from build123d import *

# Parameters (mm, degrees)
SKETCH1_W   = 40
SKETCH1_H   = 40
SKETCH1_W_2 = 32
SKETCH1_H_2 = 32


with BuildPart() as part:
    # Sweep1: sweep along a curve in space
    with BuildLine() as sweep1_path:
        add(Edge.make_bspline(
            [(0, 0, -520), (0, 0, 520)],
            knots=[0, 0, 1, 1], degree=1))
    # Sketch1 → Sweep1 (sweep)
    with BuildSketch(Plane.XY):
        Rectangle(SKETCH1_W, SKETCH1_H)
        Rectangle(SKETCH1_W_2, SKETCH1_H_2, mode=Mode.SUBTRACT)
    sweep(path=sweep1_path.line)


solid = part.part
Design review of the part built by this model. Coordinates are the model's own, in mm. A direction names the side the tool comes from. Round coordinates to 2 decimals unless told otherwise and drop trailing zeros. Loops run counter-clockwise (first coordinate to the right, second up) from the corner with the lowest first, then second, coordinate; pieces in that order, holes last. Notation, with made-up numbers: (55.5, 39.25) -> (70.5, 39.25) arc R29 cw to (70.5, 59.25) -> close; hole circle Ø11 at (9, 45.5). An arc over 180 degrees is marked (long way). Use one line per item in the form item = value. Start each with the question number.
Q1. We need section C-C on z = -377.5. Give the boundary of the cut face in (x, y).
Q2. For pin 1 Ø12 at (x, y) = (12, 13.5) entering from +Z, flat-tipped, find the tip position at first contact; note if it passes through.
Q3. Wall thickness on line 1 along Y through (x, z) = (5, 251): over which ranges is the line inside the solid? List them lowest first. Write a range as [from, to].
Q4. Draft analysis for pull direction Y (two halves, no side actions). For faces 3 (the face through (0, -16, 7)), 4 (the face through (-18, 0, -520)), 5 (the face through (0, 20, 7)), state which applies: +Y half, -Y half, draft (parallel to the pull), parting line (faces both ways), or undercut.
Q5. Machinability: for faces 1 (the face through (-16, 0, 7)), 2 (the face through (0, -20, 7)), which of the approach directions +Z, -Z, +X, -X, +Y, -Y give a long, thin tool a straight path to every point of the face, cutting with its end or side? Answer none if there is none.
Q6. We need section A-A on x = -7. Give the boundary of the cut face in (y, z).
Calculated:
q1.outline = (-20, -20) -> (20, -20) -> (20, 20) -> (-20, 20) -> close; hole (-16, -16) -> (16, -16) -> (16, 16) -> (-16, 16) -> close
q2.pin_1 = 520
q3.line_1 = [-20, -16], [16, 20]
q4.face_3 = undercut
q4.face_4 = draft
q4.face_5 = +Y half
q5.face_1 = +Z, -Z
q5.face_2 = +Z, -Z, +X, -X, -Y
q6.outline = (-20, -520) -> (-16, -520) -> (-16, 520) -> (-20, 520) -> close; (16, -520) -> (20, -520) -> (20, 520) -> (16, 520) -> close
